Design review of the part built by this model. Coordinates are the model's own, in mm. A direction names the side the tool comes from. Give positions to 0.01 mm unless a question says otherwise; leave off trailing zeros. Order: outer loops, then holes, each group sorted by start corner. A loop starts at its lowest first (then second) coordinate and runs counter-clockwise, first axis right, second up. Notation, with made-up numbers: (21.25, 74.5) -> (58.25, 74.5) arc R20 cw to (58.25, 90.5) -> close; hole circle Ø2 at (9.5, -29.75). An arc over 180 degrees is marked (long way). One line per item, written item: value. Start each with the question number.
1) Consider section A-A (z = -2.5). State the section outline as (x, y) points.
2) Wall thickness on line 1 along Z through (x, y) = (6.8, 2.5); line 2 along Z through (x, y) = (5.25, 3); line 3 along Y through (x, z) = (8, -2.5): over which ranges is each line inside the solid? List them lowest first. Write a range as from..to.
3) For pin 1 (0.9 mm diameter, centred on y = 4, z = -5, fed in from -X); pin 2 (1.3 mm diameter, centred on x = 2.5, z = -3.5, fed in from +Y); pin 3 (1.8 mm diameter, centred on y = 2.5, z = -2.5, fed in from +X), all flat-tipped, find the tip position at first contact; note any pin that passes through.
4) The part is to be moulded in two halves that separate along Y. For faces 4 (the face through (7.3, 2.5, -1.5)), 5 (the face through (6, 2, -10)), 6 (the face through (7, 5, -5)), say which applies: released by +Y, released by -Y, zero draft, split by the parting line, or undercut.
5) Tool access review of faces 1 (the face through (6, 2, 0)), 2 (the face through (4.5, 4, -5)), 3 (the face through (7.3, 2.5, -6.5)): name each direction out of +Z, -Z, +X, -X, +Y, -Y from which nothing blocks a thin tool from reaching the whole face with its end or side.
6) Consider section C-C (x = 8). State the section outline as (y, z) points, plus the area to 3 significant figures.
7) Consider section D-D (z = -8.75). State the section outline as (x, y) points, plus the area to 3 significant figures.
8) Consider section B-B (y = 2.5). State the section outline as (x, z) points.
Autodesk Inventor part; units mm, degrees
ref_plane "YZ Plane" through (0, 0, 0) normal (1, 0, 0) x (0, 1, 0)
ref_plane "XZ Plane" through (0, 0, 0) normal (0, 1, 0) x (-1, 0, 0)
ref_plane "XY Plane" through (0, 0, 0) normal (0, 0, 1) x (1, 0, 0)
sketch "Sketch1" plane through (0, 0, 0) normal (1, 0, 0) x (0, 1, 0)
  line L0 (0, 0) -> (5, 0)
  line L1 (5, 0) -> (5, -10)
  line L2 (5, -10) -> (0, -10)
  line L3 (0, -10) -> (0, 0)
  dimension "d0" = 5
  dimension "d1" = 10
extrude "Extrusion1" add sketch "Sketch1" along normal blind 10
sketch "Sketch2" plane through (0, 5, 0) normal (0, 1, 0) x (1, 0, 0)
  line L0 (0, 0) -> (10, 0)
  line L1 (0, 10) -> (10, 10)
  line L2 (10, 0) -> (6.5, 0)
  line L3 (6.5, 0) -> (6.5, 10)
  line L4 (6.5, 10) -> (10, 10)
  line L5 (10, 10) -> (10, 0)
  line L6 (6.5, 0) -> (4.5, 0)
  line L7 (4.5, 0) -> (4.5, 10)
  line L8 (4.5, 10) -> (6.5, 10)
  line L9 (6.5, 10) -> (6.5, 0)
  line L10 (4.5, 10) -> (2, 10)
  line L11 (2, 10) -> (2, 0)
  line L12 (2, 0) -> (4.5, 0)
  line L13 (4.5, 0) -> (4.5, 10)
  line L14 (0, 10) -> (0, 0)
  line L15 (2, 0) -> (0, 0)
  line L16 (0, 0) -> (0, 10)
  line L17 (0, 10) -> (2, 10)
  line L18 (2, 10) -> (2, 0)
  dimension "d4" = 3.5
  dimension "d5" = 2
  dimension "d6" = 2.5
extrude "Extrusion2" cut sketch "Sketch2" against normal blind 3 contours L14 L1 L11 L0 | L11 L1 L7 L0
sketch "Sketch3" plane through (10, 0, 0) normal (1, 0, 0) x (0, 0, -1)
  line L0 (10, 5) -> (0, 5)
  line L1 (0, 5) -> (2.5, 5)
  line L2 (2.5, 5) -> (2.5, 2.5)
  line L3 (2.5, 2.5) -> (0, 2.5)
  line L4 (0, 2.5) -> (0, 5)
  line L5 (10, 5) -> (7.5, 5)
  line L6 (7.5, 5) -> (7.5, 2.5)
  line L7 (7.5, 2.5) -> (10, 2.5)
  line L8 (10, 2.5) -> (10, 5)
  circle A0 centre (2.5, 2.5) radius 1
  circle A1 centre (7.5, 2.5) radius 1
  point P0 (0, 0)
  dimension "d9" = 2.5
  dimension "d10" = 2.5
  dimension "d11" = 2.5
  dimension "d12" = 2.5
  dimension "d13" = 2
  dimension "d14" = 2
extrude "Extrusion3" cut sketch "Sketch3" against normal blind 5.5 contours A1 L7 L6 | L6 L7 A1 | A0 L3 L2 | L2 L3 A0
properties part number "suport2_pcb_temp"
Checked values:
1. outline: (0, 0) -> (10, 0) -> (10, 1.5) -> (4.5, 1.5) -> (4.5, 2) -> (0, 2) -> close; (4.5, 3.5) -> (10, 3.5) -> (10, 5) -> (4.5, 5) -> close
2. line 1: z = -10..-8.5, -6.5..-3.5, -1.5..0
2. line 2: z = -10..-8.37, -6.63..-3.37, -1.63..0
2. line 3: y = 0..1.5, 3.5..5
3. pin 1: stops at x = 4.5
3. pin 2: stops at y = 2
3. pin 3: stops at x = 4.5
4. face 4: undercut
4. face 5: zero draft
4. face 6: released by +Y
5. face 1: +Z, +X, -X, +Y, -Y
5. face 2: +Z, -Z, -X, +Y
5. face 3: +X
6. outline: (0, -10) -> (5, -10) -> (5, 0) -> (0, 0) -> close; hole circle Ø2 at (2.5, -7.5); hole circle Ø2 at (2.5, -2.5)
6. area: 43.7 mm^2
7. outline: (0, 0) -> (10, 0) -> (10, 5) -> (4.5, 5) -> (4.5, 2) -> (0, 2) -> close
7. area: 36.5 mm^2
8. outline: (4.5, -10) -> (10, -10) -> (10, -8.5) -> (4.5, -8.5) -> close; (4.5, -6.5) -> (10, -6.5) -> (10, -3.5) -> (4.5, -3.5) -> close; (4.5, -1.5) -> (10, -1.5) -> (10, 0) -> (4.5, 0) -> close
